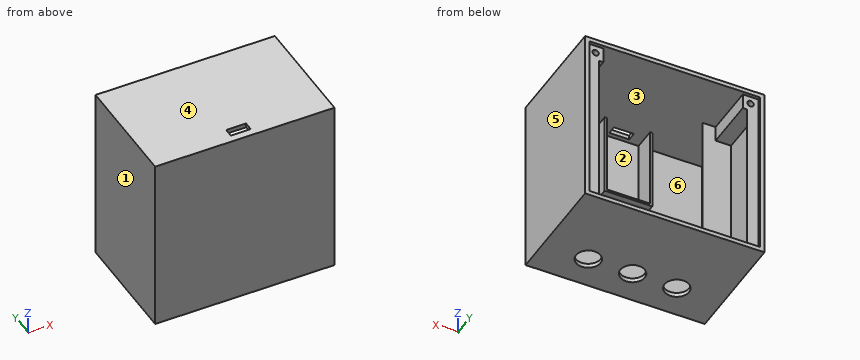
Autodesk Inventor part; units mm, degrees
ref_plane "YZ Plane" through (0, 0, 0) normal (1, 0, 0) x (0, 1, 0)
ref_plane "XZ Plane" through (0, 0, 0) normal (0, 1, 0) x (-1, 0, 0)
ref_plane "XY Plane" through (0, 0, 0) normal (0, 0, 1) x (1, 0, 0)
sketch "Sketch1" plane through (0, 0, 0) normal (0, 1, 0) x (-1, 0, 0)
  line L0 (40.5, 40.5) -> (-40.5, 40.5)
  line L1 (-40.5, 40.5) -> (-40.5, -40.5)
  line L2 (-40.5, -40.5) -> (40.5, -40.5)
  line L3 (40.5, -40.5) -> (40.5, 40.5)
  line L4 (40.5, 40.5) -> (-40.5, -40.5) construction
  line L5 (-40.5, 40.5) -> (40.5, -40.5) construction
  point P0 (0, 0)
  dimension "box_width" = 81
  dimension "box_height" = 81
extrude "Base" add sketch "Sketch1" against normal blind 1.5
sketch "Sketch2" plane through (0, 0, 0) normal (0, 1, 0) x (-1, 0, 0)
  line L0 (40.5, -40.5) -> (-40.5, -40.5)
  line L1 (40.5, 40.5) -> (-40.5, 40.5)
  line L2 (-40.5, 40.5) -> (-40.5, -40.5)
  line L3 (-40.5, -40.5) -> (40.5, -40.5)
  line L4 (40.5, -40.5) -> (40.5, 40.5)
  line L5 (40.5, 40.5) -> (-40.5, -40.5) construction
  line L6 (-40.5, 40.5) -> (40.5, -40.5) construction
  line L7 (38.5, 38.5) -> (-38.5, 38.5)
  line L8 (-38.5, 38.5) -> (-38.5, -38.5)
  line L9 (-38.5, -38.5) -> (38.5, -38.5)
  line L10 (38.5, -38.5) -> (38.5, 38.5)
  line L11 (38.5, 38.5) -> (-38.5, -38.5) construction
  line L12 (-38.5, 38.5) -> (38.5, -38.5) construction
  point P0 (0, 0)
  dimension "wall_thickness" = 2
extrude "Wall" add sketch "Sketch2" along normal blind 50
sketch "Sketch3" plane through (0, 0, 0) normal (0, 1, 0) x (-1, 0, 0)
  line L0 (-9.75, 39.5) -> (9.75, 39.5)
  line L1 (9.75, 39.5) -> (9.75, 1.7)
  line L2 (9.75, 1.7) -> (-9.75, 1.7)
  line L3 (-9.75, 1.7) -> (-9.75, 39.5)
  line L4 (-9.75, 39.5) -> (9.75, 1.7) construction
  line L5 (9.75, 39.5) -> (-9.75, 1.7) construction
  line L6 (0, 20.6) -> (0, 0) construction
  line L7 (10.75, 40.5) -> (-10.75, 40.5)
  line L8 (-10.75, 40.5) -> (-10.75, 0.7)
  line L9 (-10.75, 0.7) -> (10.75, 0.7)
  line L10 (10.75, 0.7) -> (10.75, 40.5)
  line L11 (10.75, 40.5) -> (-10.75, 0.7) construction
  line L12 (-10.75, 40.5) -> (10.75, 0.7) construction
  line L13 (40.5, 40.5) -> (-40.5, 40.5)
  point P0 (0, 40.5)
  dimension "d7" = 37.8
  dimension "d8" = 19.5
  dimension "d9" = 1
  dimension "d10" = 1
extrude "Teensy Wall" add sketch "Sketch3" along normal blind 10
sketch "Sketch4" plane through (40.5, -1.5, -40.5) normal (0, 0, -1) x (-1, 0, 0)
  line L0 (79, 51.5) -> (2, 51.5) construction
  line L1 (2, 51.5) -> (79, 51.5) construction
  line L2 (40.5, 51.5) -> (40.5, 15) construction
  line L3 (40.5, 15) -> (20.5, 15) construction
  circle A0 centre (20.5, 15) radius 5.5
  line L4 (40.5, 15) -> (40.5, 0) construction
  line L5 (81, 0) -> (0, 0) construction
  circle A1 centre (40.5, 15) radius 5.5
  circle A2 centre (60.5, 15) radius 5.5
  dimension "d21" = 11
  dimension "d23" = 20
  dimension "d59" = 20
extrude "BNC Holes" cut sketch "Sketch4" against normal up to surface (2 mm away)
sketch "Sketch7" plane through (-38.5, 0, -38.5) normal (0, 0, 1) x (1, 0, 0)
  line L0 (79, 50) -> (-2, 50)
  line L1 (-2, -1.5) -> (-2, 50)
  line L2 (-2, 50) -> (-2, 25) construction
  line L3 (-2, 25) -> (13, 25)
  line L4 (13, 25) -> (-2, 15)
  line L5 (-2, 15) -> (-2, 25)
  line L6 (38.5, 50) -> (38.5, 0) construction
  line L7 (79, -1.5) -> (79, 50)
  line L8 (79, 50) -> (79, 25) construction
  line L9 (79, 25) -> (64, 25)
  line L10 (64, 25) -> (79, 15)
  line L11 (79, 15) -> (79, 25)
  point P0 (-2, 30)
  dimension "d32" = 25
  dimension "d33" = 10
  dimension "d34" = 15
extrude "Battery Support" add sketch "Sketch7" along normal up to next
sketch "Sketch8" plane through (-40.5, -1.5, 40.5) normal (0, 0, 1) x (1, 0, 0)
  line L0 (79, 51.5) -> (2, 51.5) construction
  line L1 (40.5, 51.5) -> (40.5, 1.5) construction
  line L2 (36, 3.5) -> (45, 3.5)
  line L3 (45, 3.5) -> (45, 7.5)
  line L4 (45, 7.5) -> (36, 7.5)
  line L5 (36, 7.5) -> (36, 3.5)
  line L6 (36, 3.5) -> (45, 7.5) construction
  line L7 (45, 3.5) -> (36, 7.5) construction
  point P0 (40.5, 5.5)
  dimension "d36" = 9
  dimension "d37" = 4
  dimension "d38" = 2
extrude "USB Hole" cut sketch "Sketch8" against normal up to next
sketch "Sketch9" plane through (-38.5, 25, -38.5) normal (0, 1, 0) x (1, 0, 0)
  line L0 (0, 0) -> (77, 0)
  line L1 (64, 0) -> (64, -77)
  line L2 (49.25, -77) -> (77, -77)
  line L3 (77, 0) -> (77, -77)
  line L4 (85.7069, 0) -> (84.513, 0)
  line L5 (77, -77) -> (70, -77)
  line L6 (70, -77) -> (70, -70)
  line L7 (70, -70) -> (77, -70)
  line L8 (77, -70) -> (77, -77)
  line L9 (77, 0) -> (0, 0)
  line L10 (0, -77) -> (5.9059, -77)
  line L11 (0, -77) -> (5.9059, -77)
  line L12 (0, -77) -> (7, -77)
  line L13 (7, -77) -> (7, -70)
  line L14 (7, -70) -> (0, -70)
  line L15 (0, -70) -> (0, -77)
  line L16 (77, -77) -> (0, -77)
  line L17 (0, -77) -> (0, 0)
  dimension "d66" = 7
extrude "Plate Support" add sketch "Sketch9" along normal blind 23.5 contours L14 L13 L12 L10 L15 | L3 L2 L6 L7
sketch "Sketch15" plane through (-38.5, 0, -38.5) normal (0, 0, 1) x (1, 0, 0)
  line L0 (-2, 48.5) -> (-2, 41.5)
  line L1 (-2, 41.5) -> (5, 48.5)
  line L2 (5, 48.5) -> (-2, 48.5)
  line L3 (-2, -1.5) -> (-2, 50)
  line L4 (79, 50) -> (-2, 50)
  line L5 (38.5, 50) -> (38.5, -1.5)
  line L6 (-2, -1.5) -> (79, -1.5)
  line L7 (79, 48.5) -> (79, 41.5)
  line L8 (79, 41.5) -> (72, 48.5)
  line L9 (72, 48.5) -> (79, 48.5)
  point P0 (38.5, 0)
  dimension "d70" = 7
  dimension "d71" = 1.5
extrude "Extrusion12" add sketch "Sketch15" along normal up to surface (79 mm away) contours L2 L1 L0 | L7 L8 L9
sketch "Sketch14" plane through (-38.5, 48.5, -38.5) normal (0, 1, 0) x (1, 0, 0)
  circle A0 centre (3.5, -73.5) radius 1.45
  line L0 (7, -70) -> (7, -77) construction
  line L1 (3.5, -73.5) -> (7, -70) construction
  line L2 (3.5, -73.5) -> (7, -77) construction
  line L3 (77, -77) -> (0, -77) construction
  line L4 (0, -77) -> (3.5, -73.5) construction
  circle A1 centre (73.5, -73.5) radius 1.45
  line L5 (70, -77) -> (70, -70) construction
  line L6 (70, -70) -> (73.5, -73.5) construction
  line L7 (70, -70) -> (77, -70) construction
  line L8 (73.5, -73.5) -> (77, -70) construction
  line L9 (73.5, -73.5) -> (70, -77) construction
  point P0 (38.5, -38.5)
  dimension "d67" = 2.9
extrude "Extrusion11" cut sketch "Sketch14" against normal blind 10
properties part number "teensy_box"
Geometry: final body of the model. Coordinates: model frame, mm. Face numbers are marked on the shaded views. A direction names the side the tool comes from. Round coordinates to 2 decimals unless told otherwise and drop trailing zeros. Order: outer loops, then holes, each group sorted by start corner. A loop starts at its lowest first (then second) coordinate and runs counter-clockwise, first axis right, second up. Notation, with made-up numbers: M -10,87 L -4,87 A16 cw -4,115 Z; hole C -22.75,49.25 d5. An arc over 180 degrees is marked long. Use one line per item in the form item = value. Start each with the question number.
Q1. Access query for the marked faces 1, 2 and 3. Directions: +Z, -Z, +X, -X, +Y, -Y. A direction counts if a zero-diameter tool reaches every point of the face in a straight line with its end or side. Return the directions, or none.
Q2. Cut plane A-A (x = 20). Return loops of the section in (y, z).
Q3. Pin query (flat end, axial travel): pin 1 Ø12 at (x, z) = (-22, 28) entering from +Y; pin 2 Ø6.5 at (x, y) = (0, 13.5) entering from -Z; pin 3 Ø6 at (x, z) = (32, 9) entering from +Y. Return the tip coordinate at first contact, or that it passes through.
Q4. Mould query, pull axis Z, two halves, no side actions, for the marked faces 4, 5 and 6. Classes: +Z half, -Z half, draft (parallel to the pull), parting line (faces both ways), or undercut.
Q5. Cut plane D-D (x = 0). Return loops of the section in (y, z).
Q6. Cut plane B-B (y = 30). Return loops of the section in (x, z).
Q7. Material intervals for line 1 (X direction, y = 42.75, z = 35); line 2 (Z direction, x = 35, y = 46.5); line 3 (X direction, y = 9.5, z = 7), sorted ascending. Write a range as [from, to].
Geometry results:
q1.face_1 = +Z, -Z, -X, +Y, -Y
q1.face_2 = +Y
q1.face_3 = none
q2.outline = M -1.5,-40.5 L 8,-40.5 L 8,-38.5 L 0,-38.5 L 0,38.5 L 50,38.5 L 50,40.5 L -1.5,40.5 Z; M 19,-40.5 L 50,-40.5 L 50,-38.5 L 19,-38.5 Z
q3.pin_1 = 25
q3.pin_2 = 38.5
q3.pin_3 = 48.5
q4.face_4 = +Z half
q4.face_5 = draft
q4.face_6 = undercut
q5.outline = M -1.5,-40.5 L 8,-40.5 L 8,-38.5 L 0,-38.5 L 0,0.7 L 10,0.7 L 10,1.7 L 0,1.7 L 0,38.5 L 2,38.5 L 2,40.5 L -1.5,40.5 Z; M 6,38.5 L 50,38.5 L 50,40.5 L 6,40.5 Z; M 19,-40.5 L 50,-40.5 L 50,-38.5 L 19,-38.5 Z
q6.outline = M -40.5,-40.5 L 40.5,-40.5 L 40.5,40.5 L -40.5,40.5 Z; hole M -38.5,-38.5 L 38.5,-38.5 L 38.5,31.5 L 31.5,31.5 L 31.5,38.5 L -31.5,38.5 L -31.5,31.5 L -38.5,31.5 Z
q7.line_1 = [-40.5, -36.45], [-33.55, -31.5], [31.5, 33.55], [36.45, 40.5]
q7.line_2 = [-40.5, -38.5], [31.5, 33.55], [36.45, 40.5]
q7.line_3 = [-40.5, -38.5], [-10.75, -9.75], [9.75, 10.75], [38.5, 40.5]
